Here's how the part is built. I have some questions about the finished solid (model axes, mm). A direction names the side the tool comes from. Round coordinates to 2 decimals unless told otherwise and drop trailing zeros. Order: outer loops, then holes, each group sorted by start corner. A loop starts at its lowest first (then second) coordinate and runs counter-clockwise, first axis right, second up. Notation, with made-up numbers: (83.25, 79) -> (142.25, 79) arc R22 ccw to (142.25, 114) -> close; hole circle Ø6 at (43.5, 73.25). An arc over 180 degrees is marked (long way). Use a Markdown table: item, result. Add a question column.
(1) I want a section at D-D, the plane z = 9. Please give me the cut outline in (x, y), then the cut area to 3 significant figures.
(2) Thinking about a two-plate mould opening in X: for faces 1 (the face through (-5.18, 3.03, 2)), 2 (the face through (-1.386, -3.19, 9.575)), 3 (the face through (5.22, 2.96, 2)), which applies, pulls with the +X half, pulls with the -X half, needs draft (parallel to the pull), parting line crosses it, or undercut?
(3) I'm going to push flat-ended pins straight in: P1, Ø3, axis at y = 5, z = 3, coming from the -X side; P2, Ø3.5, axis at x = 0, z = 9, coming from the +Y side; P3, Ø2, axis at y = -0.5, z = 10, coming from the +X side. Where does each tip first touch, or does it pass through?
(4) I want a section at A-A, the plane z = 1.5. Please give me the cut outline in (x, y).
(5) I want a section at B-B, the plane y = 0. Please give me the cut outline in (x, z), then the cut area to 3 significant figures.
(6) I want a section at C-C, the plane x = 0. Please give me the cut outline in (y, z).
(7) If I drill on probe 1 along Z at (x, y) = (0, 2.8); probe 2 along Y at (x, z) = (-1, 10.75); probe 3 along X at (y, z) = (1.25, 9.25), over which ranges is the centre line in solid material (lowest first)?
(8) On a 3-axis mill with a long thin cutter (end or side, diameter ignored), from which of +Z, -Z, +X, -X, +Y, -Y can I reach the whole of each face in a straight line? I mean faces 4 (the face through (-4, -4, 4)), 5 (the face through (0, -6, 2)). Say none if no direction works.
from build123d import *

# Parameters (mm, degrees)
BOSS_EXTRUDE1_DEPTH   = 4
SKETCH2_R             = 5
BOSS_EXTRUDE2_DEPTH   = 10
SKETCH3_R             = 2
CUT_EXTRUDE1_DEPTH    = 15
F_3_0MM_DOWEL_SLOT5_D = 3
FILLET1_R             = 0.5


with BuildPart() as part:
    # Sketch1 → Boss-Extrude1 (new body)
    with BuildSketch(Plane.XY):
        with BuildLine():
            Line((-2.886751346, -6), (2.886751346, -6))
            ThreePointArc((2.886751346, -6), (3.386751346, -5.866025404), (3.75277675, -5.5))
            Line((3.75277675, -5.5), (6.639528096, -0.5))
            ThreePointArc((6.639528096, -0.5), (6.773502692, 0), (6.639528096, 0.5))
            Line((6.639528096, 0.5), (3.75277675, 5.5))
            ThreePointArc((3.75277675, 5.5), (3.386751346, 5.866025404), (2.886751346, 6))
            Line((2.886751346, 6), (-2.886751346, 6))
            ThreePointArc((-2.886751346, 6), (-3.386751346, 5.866025404), (-3.75277675, 5.5))
            Line((-3.75277675, 5.5), (-6.639528096, 0.5))
            ThreePointArc((-6.639528096, 0.5), (-6.773502692, 0), (-6.639528096, -0.5))
            Line((-6.639528096, -0.5), (-3.75277675, -5.5))
            ThreePointArc((-3.75277675, -5.5), (-3.386751346, -5.866025404), (-2.886751346, -6))
        make_face()
    extrude(amount=BOSS_EXTRUDE1_DEPTH)

    # Sketch2 → Boss-Extrude2 (add)
    with BuildSketch(Plane.XY.offset(4)):
        Circle(SKETCH2_R)
    extrude(amount=BOSS_EXTRUDE2_DEPTH)

    # Sketch3 → Cut-Extrude1 (cut, through all)
    with BuildSketch(Plane.XY.offset(14)):
        Circle(SKETCH3_R)
    extrude(amount=-CUT_EXTRUDE1_DEPTH, mode=Mode.SUBTRACT)

    # Ø3.0mm Dowel Slot5 (through all)
    with Locations(Plane(origin=(0, 6, 0), x_dir=(1, 0, 0), z_dir=(0, 1, 0))):
        with Locations((0, -9)):
            Hole(F_3_0MM_DOWEL_SLOT5_D / 2)

    # Fillet1
    fillet1_edges = [part.edges().sort_by_distance(p)[0] for p in [
        (-5, 0, 14),
    ]]
    fillet(fillet1_edges, radius=FILLET1_R)

    # Sketch12 → Cut-Revolve1 (revolve, cut)
    with BuildSketch(Plane(origin=(0, 0, 0), x_dir=(1, 0, 0), z_dir=(0, 1, 0))):
        Polygon((0, 0), (0, -0.526706506), (-1.691943312, -0.526706506), (-3.449696503, 0.470605478), (-4.989422791, 0.470605478), (-6.968108857, -0.553510453), (-7.302945228, -0.553510453), (-7.302945228, 1.336347729), (0, 1.336347729), align=None)
    revolve(axis=Axis((0, 0, -3.230240026), (0, 0, 1)), mode=Mode.SUBTRACT)


solid = part.part
Taken from the geometry:
| question | item | result |
|---|---|---|
| 1 | outline | (-1.5, -4.77) -> (-1.5, -1.32) arc R2 cw to (-1.5, 1.32) -> (-1.5, 4.77) arc R5 ccw to start; (1.5, -4.77) arc R5 ccw to (1.5, 4.77) -> (1.5, 1.32) arc R2 cw to (1.5, -1.32) -> close |
| 1 | area | 47.2 mm2 |
| 2 | face 1 | pulls with the -X half |
| 2 | face 2 | undercut |
| 2 | face 3 | pulls with the +X half |
| 3 | P1 | stops at x = -4.91 |
| 3 | P2 | stops at y = 5 |
| 3 | P3 | stops at x = 5 |
| 4 | outline | (-6.64, -0.5) -> (-3.75, -5.5) arc R1 ccw to (-2.89, -6) -> (2.89, -6) arc R1 ccw to (3.75, -5.5) -> (6.64, -0.5) arc R1 ccw to (6.64, 0.5) -> (3.75, 5.5) arc R1 ccw to (2.89, 6) -> (-2.89, 6) arc R1 ccw to (-3.75, 5.5) -> (-6.64, 0.5) arc R1 ccw to start; hole circle Ø4 at (0, 0) |
| 5 | outline | (-6.77, 0.45) -> (-5.9, 0) -> (-2.62, 0) -> (-2, 0.35) -> (-2, 14) -> (-4.5, 14) arc R0.5 ccw to (-5, 13.5) -> (-5, 4) -> (-6.77, 4) -> close; (2, 0.35) -> (2.62, 0) -> (5.9, 0) -> (6.77, 0.45) -> (6.77, 4) -> (5, 4) -> (5, 13.5) arc R0.5 ccw to (4.5, 14) -> (2, 14) -> close |
| 5 | area | 97.5 mm2 |
| 6 | outline | (-6, 0.05) -> (-5.9, 0) -> (-2.62, 0) -> (-2, 0.35) -> (-2, 7.5) -> (-5, 7.5) -> (-5, 4) -> (-6, 4) -> close; (-5, 10.5) -> (-2, 10.5) -> (-2, 14) -> (-4.5, 14) arc R0.5 ccw to (-5, 13.5) -> close; (2, 0.35) -> (2.62, 0) -> (5.9, 0) -> (6, 0.05) -> (6, 4) -> (5, 4) -> (5, 7.5) -> (2, 7.5) -> close; (2, 10.5) -> (5, 10.5) -> (5, 13.5) arc R0.5 ccw to (4.5, 14) -> (2, 14) -> close |
| 7 | probe 1 | z = 0 to 7.5, 10.5 to 14 |
| 7 | probe 2 | y = -4.9 to -1.73, 1.73 to 4.9 |
| 7 | probe 3 | x = -4.84 to -1.56, 1.56 to 4.84 |
| 8 | face 4 | +Z |
| 8 | face 5 | +Z, -Z, +X, -X, -Y |
